Check sheet for the modelled part. Datum: model origin and axes. Units: mm. Face numbers are marked on the shaded views. A direction names the side the tool comes from. Coordinates: 2 decimals unless noted, no trailing zeros. Loops run counter-clockwise (first coordinate to the right, second up) from the corner with the lowest first, then second, coordinate; pieces in that order, holes last.
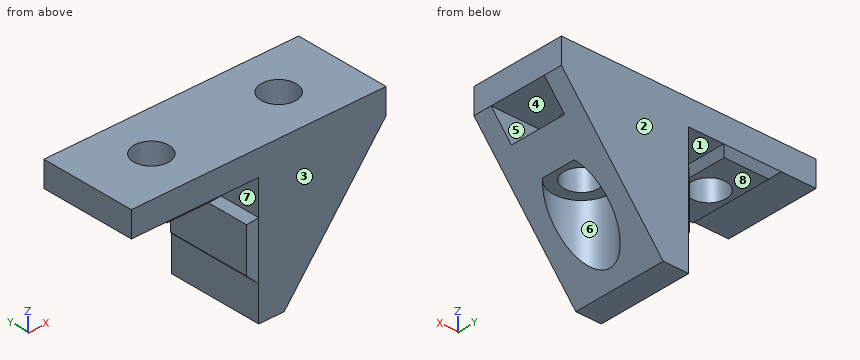
```python
from build123d import *

# Parameters (mm, degrees)
F0_W      = 40
F0_H      = 15
F1_DEPTH  = 4
F2_W      = 9
F2_H      = 15
F2_W_2    = 4
F3_DEPTH  = 1
F4_DEPTH  = 19
F5_W      = 15
F5_H      = 9
F6_DEPTH  = 1
F7_SIZE   = 0.99999
F9_DEPTH  = 15
F12_DEPTH = 4
F13_R     = 2.75
F14_DEPTH = 24.001
F15_R     = 4.5
F16_DEPTH = 12


# Not quite as in the source:
# - a fillet or chamfer is up to 0.001 mm smaller than in the source, because OpenCascade refuses the exact size


with BuildPart() as f1:
    # F0 (on Top) → F1 (new body)
    with BuildSketch(Plane.XY):
        with Locations((20, 7.5)):
            Rectangle(F0_W, F0_H)
    extrude(amount=F1_DEPTH)

    # F2 (on face) → F3 (join)
    with BuildSketch(Plane(origin=(0, 0, 0), x_dir=(1, 0, 0), z_dir=(0, 0, -1))):
        with Locations((10, -7.5)):
            Rectangle(F2_W, F2_H)
        with Locations((22, -7.5)):
            Rectangle(F2_W_2, F2_H)
    extrude(amount=F3_DEPTH)

    # F4 (add): a face of the model
    f4_faces = [f1.faces().sort_by_distance(p)[0] for p in [
        (22, 7.5, -1),
    ]]
    extrude(f4_faces, amount=F4_DEPTH)

    # F5 (on face) → F6 (join)
    with BuildSketch(Plane(origin=(20, 0, 0), x_dir=(0, -1, 0), z_dir=(-1, 0, 0))):
        with Locations((-7.5, -10)):
            Rectangle(F5_W, F5_H)
    extrude(amount=F6_DEPTH)

    # F7 (size 1 in the source; OpenCascade refuses exactly that, so slightly less here)
    f7_edges = [f1.edges().sort_by_distance(p)[0] for p in [
        (19, 15, -10),
        (19, 7.5, -14.5),
        (19, 0, -10),
        (19, 7.5, -5.5),
        (10, 0, -1),
        (5.5, 7.5, -1),
        (10, 15, -1),
        (14.5, 7.5, -1),
    ]]
    chamfer(f7_edges, length=F7_SIZE)

    # F8 (on face) → F9 (join, through all)
    with BuildSketch(Plane.XZ):
        Polygon((40, 0), (24, 0), (24, -20), align=None)
    extrude(amount=-F9_DEPTH)

    # F11 (on offset) → F12 (cut)
    with BuildSketch(Plane.XY):
        Polygon((26.05, 5.2194664367), (30, 2.9389328734), (40, 2.9389328734), (40, 12.0610671266), (30, 12.0610671266), (26.05, 9.7805335633), align=None)
    extrude(amount=-F12_DEPTH, mode=Mode.SUBTRACT)

    # F13 (on face) → F14 (cut, through all)
    with BuildSketch(Plane.XY.offset(4)):
        with Locations((30, 7.5)):
            Circle(F13_R)
        with Locations((10, 7.5)):
            Circle(F13_R)
    extrude(amount=-F14_DEPTH, mode=Mode.SUBTRACT)

    # F15 (on face) → F16 (cut)
    with BuildSketch(Plane(origin=(0, 0, -20), x_dir=(1, 0, 0), z_dir=(0, 0, -1))):
        with Locations((30, -7.5)):
            Circle(F15_R)
    extrude(amount=-F16_DEPTH, mode=Mode.SUBTRACT)


solid = f1.part
```
1) Mould release check, pull along Y, two halves, no side actions. Record for the marked faces 1, 2, 3 and 4: +Y half, -Y half, draft (parallel to the pull), parting line (faces both ways), or undercut.
Answer sheet:
face 1: draft
face 2: +Y half
face 3: -Y half
face 4: undercut
2) Section check C-C on y = 7.5. Give the number of separate pieces and of enclosed holes in the cut face, plus the area to 3 significant figures.
Answer sheet:
separate pieces: 4
enclosed holes: 0
area: 254 mm2
3) Section check A-A on x = 10. Enter the section's corners in (y, z).
Answer sheet:
outline: (0, 0) - (1, -1) - (4.75, -1) - (4.75, 4) - (0, 4) - close; (10.25, -1) - (14, -1) - (15, 0) - (15, 4) - (10.25, 4) - close
4) Section check D-D on z = -8.5. Enter the section's corners in (x, y), plus the area to 3 significant figures.
Answer sheet:
outline: (19, 1) - (20, 0) - (33.2, 0) - (33.2, 4.34) arc R4.5 cw (long way) to (33.2, 10.66) - (33.2, 15) - (20, 15) - (19, 14) - close
area: 154 mm2
5) Depth check by flat-ended pin: pin 1 (4.5 mm diameter, centred on x = 35, z = -2.5, fed in from -Y); pin 2 (6 mm diameter, centred on y = 1.5, z = -15, fed in from +X); pin 3 (1.6 mm diameter, centred on y = 8, z = -2, fed in from -X); pin 4 (2.5 mm diameter, centred on x = 29, y = 6, fed in from -Z). Enter the tip coordinate at first touch or a pass-through.
Answer sheet:
pin 1: stops at y = 0
pin 2: stops at x = 30.4
pin 3: stops at x = 20
pin 4: stops at z = -8
6) Section check B-B on z = 1. Enter the section's corners in (x, y), plus the area to 3 significant figures.
Answer sheet:
outline: (0, 0) - (40, 0) - (40, 15) - (0, 15) - close; hole circle Ø5.5 at (10, 7.5); hole circle Ø5.5 at (30, 7.5)
area: 552 mm2
7) Scan lines: line 1 (Y direction, x = 30, z = -6.75); line 2 (X direction, y = 6.5, z = 2); line 3 (X direction, y = 7.5, z = -11.25). Record each from-to range of solid material in increasing order.
Answer sheet:
line 1: y = 0 to 4.75, 10.25 to 15
line 2: x = 0 to 7.44, 12.56 to 27.44, 32.56 to 40
line 3: x = 19 to 25.5
8) Set-up check for the marked faces 5, 6, 7 and 8: record each of +Z, -Z, +X, -X, +Y, -Y from which the full face is reachable in a straight line by a thin tool's end or side.
Answer sheet:
face 5: +X
face 6: -Z
face 7: +Y, -Y
face 8: -Z, -X, +Y, -Y
